Model file for the job. Use its own axes, mm. Face numbers are marked on the shaded views. Round coordinates to 2 decimals unless told otherwise and drop trailing zeros. Loops run counter-clockwise (first coordinate to the right, second up) from the corner with the lowest first, then second, coordinate; pieces in that order, holes last.
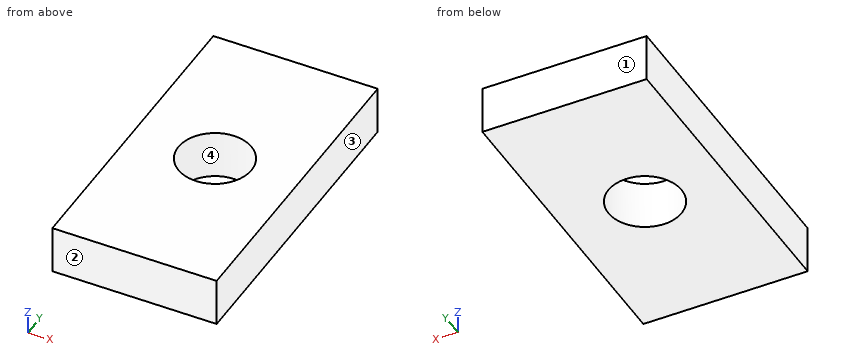
from build123d import *

# Parameters (mm, degrees)
SKETCH1_W           = 40.5
SKETCH1_H           = 76.5
BOSS_EXTRUDE1_DEPTH = 12
CUT_EXTRUDE1_REACH  = 14
SKETCH2_R           = 9


with BuildPart() as part:
    # Sketch1 → Boss-Extrude1 (new body)
    with BuildSketch(Plane.XY):
        Rectangle(SKETCH1_W, SKETCH1_H)
    extrude(amount=BOSS_EXTRUDE1_DEPTH)

    # Sketch2 → Cut-Extrude1 (cut, up to next)
    with BuildSketch(Plane.XY.offset(12), mode=Mode.PRIVATE) as cut_extrude1_sk1:
        Circle(SKETCH2_R)
    cut_extrude1_tool1 = extrude(cut_extrude1_sk1.sketch, amount=-CUT_EXTRUDE1_REACH, mode=Mode.PRIVATE) & part.part
    add(cut_extrude1_tool1.solids().sort_by_distance((0, 0, 12))[0], mode=Mode.SUBTRACT)


solid = part.part
Q1. Slice it at B-B on y = 0. Give the cut face in (x, z).
Q2. Slice it at A-A on x = 0. Give the cut face in (y, z).
Q3. Pull direction Y, two halves, no side cores. Call the marked faces 1, 2, 3 and 4: pulls with the +Y half, pulls with the -Y half, needs draft (parallel to the pull), parting line crosses it, or undercut.
Q4. Flat gauge pin, fed straight in: P1, Ø8, axis at x = 0.5, y = 9.5, coming from the -Z side. Where does the tip first touch, or does it go through?
Q5. Probe line 1 (Y direction, x = 0, z = 3.25); line 2 (Y direction, x = -2, z = 10); line 3 (X direction, y = -5, z = 9.25). List the from-to ranges inside material, lowest first.
Q6. Slice it at C-C on z = 8.25. Give the cut face in (x, y).
Reply:
1. outline: (-20.25, 0) - (-9, 0) - (-9, 12) - (-20.25, 12) - close; (9, 0) - (20.25, 0) - (20.25, 12) - (9, 12) - close
2. outline: (-38.25, 0) - (-9, 0) - (-9, 12) - (-38.25, 12) - close; (9, 0) - (38.25, 0) - (38.25, 12) - (9, 12) - close
3. face 1: pulls with the +Y half
3. face 2: pulls with the -Y half
3. face 3: needs draft
3. face 4: undercut
4. P1: stops at z = 0
5. line 1: y = -38.25 to -9, 9 to 38.25
5. line 2: y = -38.25 to -8.77, 8.77 to 38.25
5. line 3: x = -20.25 to -7.48, 7.48 to 20.25
6. outline: (-20.25, -38.25) - (20.25, -38.25) - (20.25, 38.25) - (-20.25, 38.25) - close; hole circle Ø18 at (0, 0)
